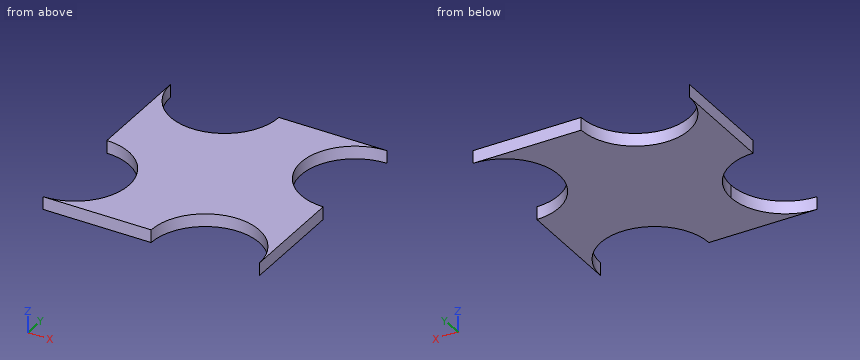
```python
from build123d import *

# Parameters (mm, degrees)
F0_W     = 101.6
F0_H     = 101.6
F1_DEPTH = 6
F3_DEPTH = 6.35


with BuildPart() as f1:
    # F0 (on Top) → F1 (new body)
    with BuildSketch(Plane.XY):
        Rectangle(F0_W, F0_H)
    extrude(amount=F1_DEPTH)

    # F2 (on face) → F3 (cut)
    with BuildSketch(Plane.XY.offset(6)):
        with BuildLine():
            ThreePointArc((-25.4, -25.4), (-32.8394877579, -7.4394877579), (-50.8, 0))
            Line((-50.8, 0), (-50.8, -50.8))
            ThreePointArc((-50.8, -50.8), (-32.8394877579, -43.3605122421), (-25.4, -25.4))
        make_face()
        with BuildLine():
            ThreePointArc((-50.8, 50.8), (-25.4, 25.4), (0, 50.8))
            Line((0, 50.8), (-50.8, 50.8))
        make_face()
        with BuildLine():
            Line((50.8, 0), (50.8, 50.8))
            ThreePointArc((50.8, 50.8), (25.4, 25.4), (50.8, 0))
        make_face()
        with BuildLine():
            Line((0, -50.8), (50.8, -50.8))
            ThreePointArc((50.8, -50.8), (25.4, -25.4), (0, -50.8))
        make_face()
    extrude(amount=-F3_DEPTH, mode=Mode.SUBTRACT)


solid = f1.part
```
Could you check a few things on this model? Use its own coordinates, in mm. Give positions to 0.01 mm unless a question says otherwise; leave off trailing zeros. Loops run counter-clockwise (first coordinate to the right, second up) from the corner with the lowest first, then second, coordinate; pieces in that order, holes last. Notation, with made-up numbers: (-13, -39) - (27, -39) arc R25 cw to (27, -24) - close; hole circle Ø6 at (46.25, 74). An arc over 180 degrees is marked (long way). Use one line per item in the form item = value.
1. I'm going to push flat-ended pins straight in: pin 1 Ø2 at (x, z) = (-15.5, 2.5) entering from +Y; pin 2 Ø3 at (y, z) = (25.5, 5) entering from +X. Where does each tip first touch, or does it pass through?
Response values:
pin_1 = 27.86
pin_2 = 25.45
2. I want a section at D-D (x = -14). Please give me the cut outline in (y, z), and give its area (3 significant figures).
Response values:
outline = (-50.8, 0) - (28.1, 0) - (28.1, 6) - (-50.8, 6) - close
area = 473 mm²
3. I want a section at B-B (x = -30). Please give me the cut outline in (y, z), and give its area (3 significant figures).
Response values:
outline = (-50.8, 0) - (-39.98, 0) - (-39.98, 6) - (-50.8, 6) - close; (-10.82, 0) - (25.82, 0) - (25.82, 6) - (-10.82, 6) - close
area = 285 mm²
4. I want a section at C-C (y = 29.5). Please give me the cut outline in (x, z).
Response values:
outline = (-50.8, 0) - (-39.24, 0) - (-39.24, 6) - (-50.8, 6) - close; (-11.56, 0) - (25.73, 0) - (25.73, 6) - (-11.56, 6) - close
5. I need wall thicknesses on probe 1 along Y at (x, z) = (24.5, 4.65); probe 2 along X at (y, z) = (-28, 0.55); probe 3 along Y at (x, z) = (45, 5.45). Which ranges of each line are inside material? Lowest first, please.
Response values:
probe_1 = -25.42 to 50.8
probe_2 = -25.53 to 14.21, 36.59 to 50.8
probe_3 = -34.64 to 0.67, 50.13 to 50.8
6. I want a section at A-A (z = 3.1). Please give me the cut outline in (x, y).
Response values:
outline = (-50.8, -50.8) - (0, -50.8) arc R25.4 cw to (50.8, -50.8) - (50.8, 0) arc R25.4 cw to (50.8, 50.8) - (0, 50.8) arc R25.4 cw to (-50.8, 50.8) - (-50.8, 0) arc R25.4 cw to start
